Job drawing, mm, ordinate dimensions from the low corner. One solid piece. A direction names the side the tool comes from. Give positions to 0.01 mm unless a question says otherwise; leave off trailing zeros. Loops run counter-clockwise (first coordinate to the right, second up) from the corner with the lowest first, then second, coordinate; pieces in that order, holes last. Notation, with made-up numbers: M -2,85.5 L 30,85.5 A20 ccw 30,122.5 Z; hole C 17,-9.75 d8. An arc over 180 degrees is marked long. Answer in a Markdown table with one row per item.
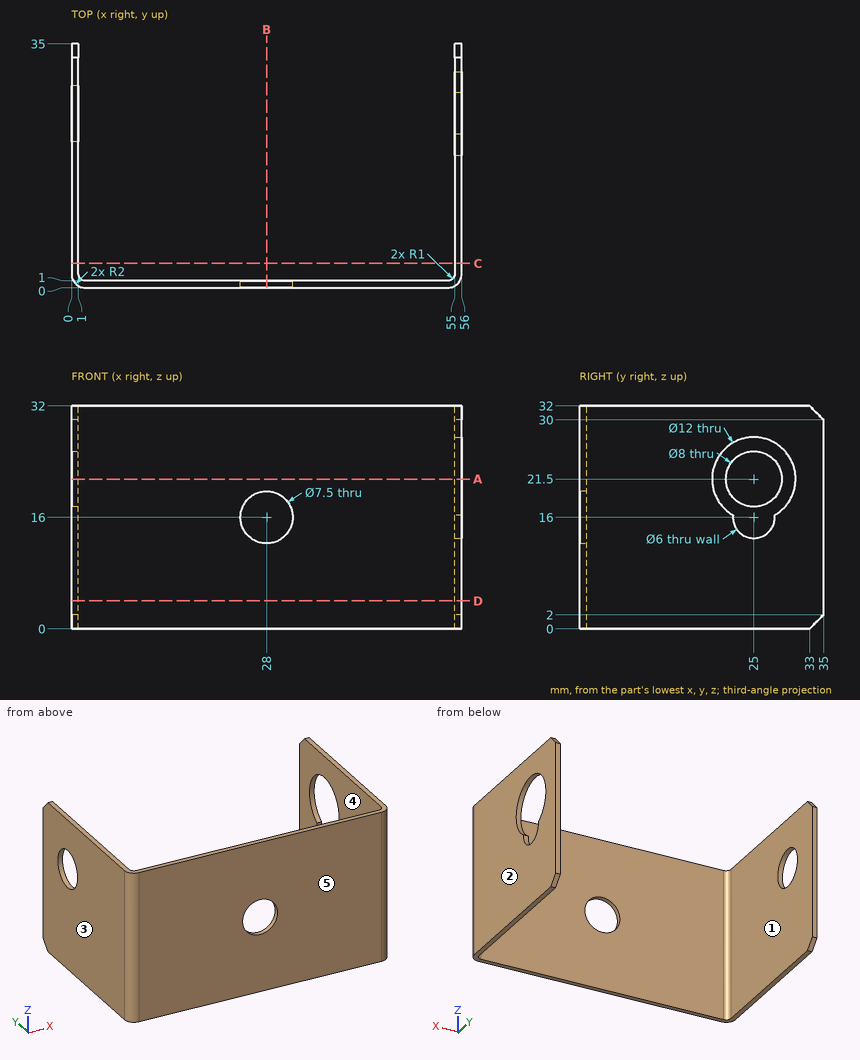
(1) Drill centre lines: line 1 along X through (y, z) = (13.5, 23); line 2 along Y through (x, z) = (6, 18). Where is each one in solid material? Low to high.
Recorded:
| item | result |
|---|---|
| line 1 | x = 0 to 1, 55 to 56 |
| line 2 | y = 0 to 1 |
(2) Saw through at A-A (z = 21.5). Write the cut outline in (x, y).
Recorded:
| item | result |
|---|---|
| outline | M 0,2 A2 ccw 2,0 L 54,0 A2 ccw 56,2 L 56,19 L 55,19 L 55,2 A1 cw 54,1 L 2,1 A1 cw 1,2 L 1,21 L 0,21 Z; M 0,29 L 1,29 L 1,35 L 0,35 Z; M 55,31 L 56,31 L 56,35 L 55,35 Z |
(3) Saw through at B-B (x = 28). Write the cut outline in (y, z).
Recorded:
| item | result |
|---|---|
| outline | M 0,0 L 1,0 L 1,12.25 L 0,12.25 Z; M 0,19.75 L 1,19.75 L 1,32 L 0,32 Z |
(4) Pull direction X, two halves, no side cores. Call the marked faces 3, 4 and 5: +X half, -X half, draft (parallel to the pull), parting line (faces both ways), or undercut.
Recorded:
| item | result |
|---|---|
| face 3 | -X half |
| face 4 | undercut |
| face 5 | draft |
(5) Pin check, flat tips, straight feed: pin 1 Ø10 at (x, y) = (50, 5.5) entering from +Z; pin 2 Ø5 at (x, z) = (7.5, 12) entering from +Y. Stop position of each tip, or through.
Recorded:
| item | result |
|---|---|
| pin 1 | stops at z = 32 |
| pin 2 | stops at y = 1 |
(6) Which spindle directions (+Z, -Z, +X, -X, +Y, -Y) get a long thin tool onto all of the face, cutting with end or side? Do the marked faces 1 and 2. Say none if no direction does.
Recorded:
| item | result |
|---|---|
| face 1 | +Z, -Z, +Y |
| face 2 | +Z, -Z, +X, +Y, -Y |
(7) Saw through at D-D (z = 4). Write the cut outline in (x, y).
Recorded:
| item | result |
|---|---|
| outline | M 0,2 A2 ccw 2,0 L 54,0 A2 ccw 56,2 L 56,35 L 55,35 L 55,2 A1 cw 54,1 L 2,1 A1 cw 1,2 L 1,35 L 0,35 Z |
(8) Saw through at C-C (y = 3.5). Write the cut outline in (x, z), plus the area to 3 significant figures.
Recorded:
| item | result |
|---|---|
| outline | M 0,0 L 1,0 L 1,32 L 0,32 Z; M 55,0 L 56,0 L 56,32 L 55,32 Z |
| area | 64.0 mm^2 |
